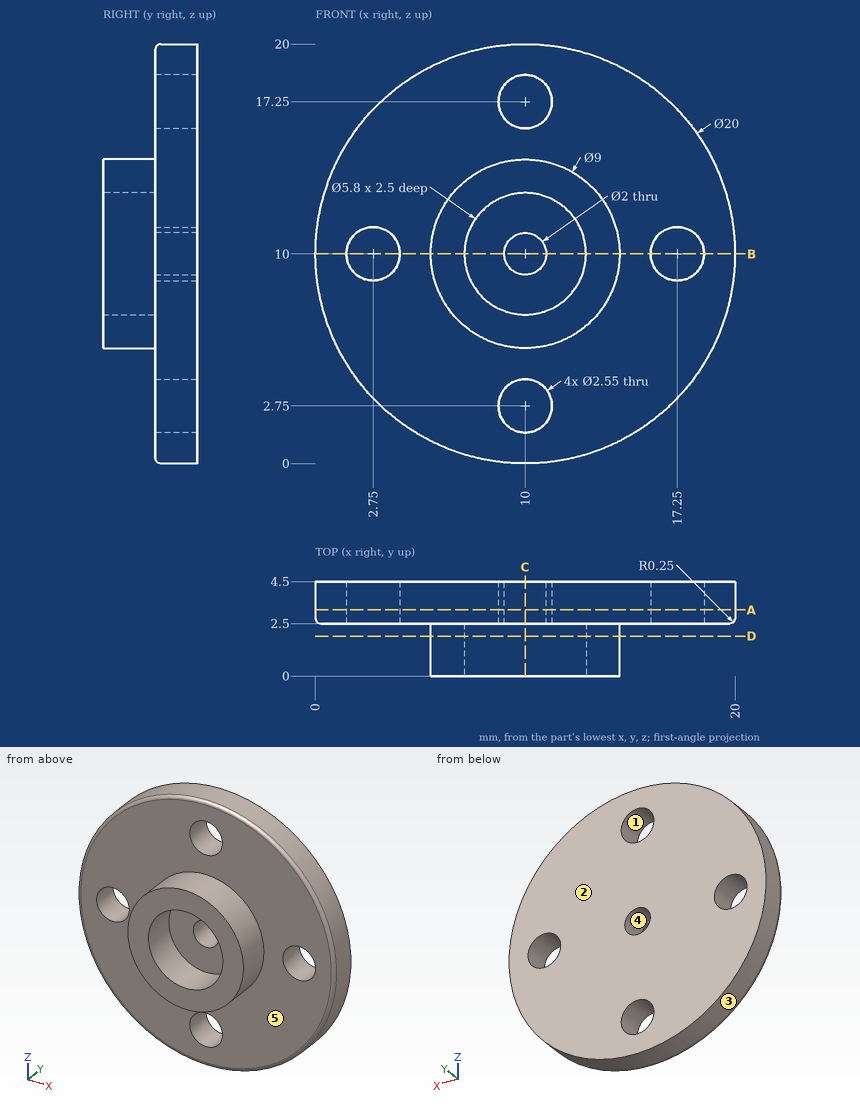
Geometry: see drawing. Coordinates: mm, zero at the bounding-box minimum. A direction names the side the tool comes from. Coordinates: 2 decimals unless noted, no trailing zeros. Loops run counter-clockwise (first coordinate to the right, second up) from the corner with the lowest first, then second, coordinate; pieces in that order, holes last.
Q1. Cut plane D-D (y = 1.9). Output: boundary loops of the cut face in (x, z), then the cut area to 3 significant figures.
Q2. Set-up query: the marked faces 4 and 5. Return all of +Z, -Z, +X, -X, +Y, -Y with unobstructed straight access to the full face (end or side cutting, diameter ignored); none if empty.
Q3. Cut plane C-C (x = 10). Output: boundary loops of the cut face in (y, z) (3 decimals), then the cut area to 3 significant figures.
Q4. Cut plane B-B (z = 10). Output: boundary loops of the cut face in (x, y) (3 decimals), then the cut area to 3 significant figures.
Q5. Contact query for flat-ended pins moving along their axis: pin 1 (1 mm diameter, centred on x = 16, y = 3.5, fed in from +Z); pin 2 (3 mm diameter, centred on x = 17.25, z = 10, fed in from -Y). Output: stop coordinate, or through.
Q6. Draft query along X for the marked faces 1, 2 and 3. Return one class per face: +X half, -X half, draft (parallel to the pull), parting line (faces both ways), or undercut.
Q7. Material intervals for line 1 (X direction, y = 3.1, z = 10) (3 decimals); line 2 (Z direction, x = 10.5, y = 4); line 3 (X direction, y = 0.95, z = 10), sorted ascending.
Q8. Cut plane A-A (y = 3.15). Output: boundary loops of the cut face in (x, z) (3 decimals).
Working result:
1. outline: circle Ø9 at (10, 10); hole circle Ø5.8 at (10, 10)
1. area: 37.2 mm2
2. face 4: +Y, -Y
2. face 5: -Y
3. outline: (0, 5.5) - (2.5, 5.5) - (2.5, 4.025) - (4.5, 4.025) - (4.5, 9) - (2.5, 9) - (2.5, 7.1) - (0, 7.1) - close; (0, 12.9) - (2.5, 12.9) - (2.5, 11) - (4.5, 11) - (4.5, 15.975) - (2.5, 15.975) - (2.5, 14.5) - (0, 14.5) - close; (2.5, 0.25) arc R0.25 ccw to (2.75, 0) - (4.5, 0) - (4.5, 1.475) - (2.5, 1.475) - close; (2.5, 18.525) - (4.5, 18.525) - (4.5, 20) - (2.75, 20) arc R0.25 ccw to (2.5, 19.75) - close
3. area: 33.8 mm2
4. outline: (0, 2.75) arc R0.25 ccw to (0.25, 2.5) - (1.475, 2.5) - (1.475, 4.5) - (0, 4.5) - close; (4.025, 2.5) - (5.5, 2.5) - (5.5, 0) - (7.1, 0) - (7.1, 2.5) - (9, 2.5) - (9, 4.5) - (4.025, 4.5) - close; (11, 2.5) - (12.9, 2.5) - (12.9, 0) - (14.5, 0) - (14.5, 2.5) - (15.975, 2.5) - (15.975, 4.5) - (11, 4.5) - close; (18.525, 2.5) - (19.75, 2.5) arc R0.25 ccw to (20, 2.75) - (20, 4.5) - (18.525, 4.5) - close
4. area: 33.8 mm2
5. pin 1: stops at z = 18.35
5. pin 2: stops at y = 2.5
6. face 1: undercut
6. face 2: draft
6. face 3: parting line
7. line 1: x = 0 to 1.475, 4.025 to 9, 11 to 15.975, 18.525 to 20
7. line 2: z = 0.01 to 1.58, 3.92 to 9.13, 10.87 to 16.08, 18.42 to 19.99
7. line 3: x = 5.5 to 7.1, 12.9 to 14.5
8. outline: circle Ø20 at (10, 10); hole circle Ø2.55 at (2.75, 10); hole circle Ø2.55 at (10, 2.75); hole circle Ø2.55 at (10, 17.25); hole circle Ø2 at (10, 10); hole circle Ø2.55 at (17.25, 10)
